For this review, take the finished solid that the model builds, in its own axes (mm). Give positions to 0.01 mm unless a question says otherwise; leave off trailing zeros. Write each loop counter-clockwise with the first axis right and the second up, starting at its lowest first coordinate (ties: lowest second). Pieces come first, ordered by that corner, then holes.
Q1. Insertion check: P1, Ø5, axis at x = 108, z = -27, coming from the -Y side; P2, Ø1.9, axis at x = -215, z = -181.4, coming from the +Y side. Each pin has a flat end and moves straight along its axis. Give the tip position at first contact, or say it passes through.
Q2. We need section A-A (x = -107.5). Write out the cut boundary in (y, z), then the cut area to 3 significant figures.
Q3. For line 1 (Z direction, x = -215, y = 0.6); line 2 (X direction, y = 0.6, z = -1.4); line 3 (X direction, y = 0.65, z = 188.6), list the stretches that pass through material, from the lowest coordinate up.
```python
from build123d import *

# Parameters (mm, degrees)
CROQUIS1_W              = 455
CROQUIS1_H              = 409
SALIENTE_EXTRUIR1_DEPTH = 1
CORTAR_EXTRUIR1_REACH   = 307.904
CROQUIS2_R              = 1.6
CORTAR_EXTRUIR2_REACH   = 307.904
CROQUIS3_R              = 5
CORTAR_EXTRUIR3_REACH   = 307.904
CROQUIS4_R              = 1.6
MOVER_CARA1_BY          = 5
CORTAR_EXTRUIR4_DEPTH   = 10


with BuildPart() as part:
    # Croquis1 → Saliente-Extruir1 (new body)
    with BuildSketch(Plane(origin=(0, 0, 0), x_dir=(1, 0, 0), z_dir=(0, 1, 0))):
        Rectangle(CROQUIS1_W, CROQUIS1_H)
    extrude(amount=SALIENTE_EXTRUIR1_DEPTH)

    # Croquis2 → Cortar-Extruir1 (cut, up to next)
    with BuildSketch(Plane.XZ, mode=Mode.PRIVATE) as cortar_extruir1_sk1:
        with Locations(Location((-215, 178.6, 0), (0, 0, 270))):
            Circle(CROQUIS2_R)
    cortar_extruir1_tool1 = extrude(cortar_extruir1_sk1.sketch, amount=-CORTAR_EXTRUIR1_REACH, mode=Mode.PRIVATE) & part.part
    # Croquis2 → Cortar-Extruir1 (cut, up to next)
    with BuildSketch(Plane.XZ, mode=Mode.PRIVATE) as cortar_extruir1_sk2:
        with Locations(Location((-215, -181.4, 0), (0, 0, 270))):
            Circle(CROQUIS2_R)
    cortar_extruir1_tool2 = extrude(cortar_extruir1_sk2.sketch, amount=-CORTAR_EXTRUIR1_REACH, mode=Mode.PRIVATE) & part.part
    # Croquis2 → Cortar-Extruir1 (cut, up to next)
    with BuildSketch(Plane.XZ, mode=Mode.PRIVATE) as cortar_extruir1_sk3:
        with Locations(Location((215, -181.4, 0), (0, 0, 270))):
            Circle(CROQUIS2_R)
    cortar_extruir1_tool3 = extrude(cortar_extruir1_sk3.sketch, amount=-CORTAR_EXTRUIR1_REACH, mode=Mode.PRIVATE) & part.part
    # Croquis2 → Cortar-Extruir1 (cut, up to next)
    with BuildSketch(Plane.XZ, mode=Mode.PRIVATE) as cortar_extruir1_sk4:
        with Locations(Location((215, 178.6, 0), (0, 0, 270))):
            Circle(CROQUIS2_R)
    cortar_extruir1_tool4 = extrude(cortar_extruir1_sk4.sketch, amount=-CORTAR_EXTRUIR1_REACH, mode=Mode.PRIVATE) & part.part
    # Croquis2 → Cortar-Extruir1 (cut, up to next)
    with BuildSketch(Plane.XZ, mode=Mode.PRIVATE) as cortar_extruir1_sk5:
        with Locations(Location((0, 31.25, 0), (0, 0, 270))):
            Circle(CROQUIS2_R)
    cortar_extruir1_tool5 = extrude(cortar_extruir1_sk5.sketch, amount=-CORTAR_EXTRUIR1_REACH, mode=Mode.PRIVATE) & part.part
    add(cortar_extruir1_tool1.solids().sort_by_distance((-215, 0, 178.6))[0], mode=Mode.SUBTRACT)
    add(cortar_extruir1_tool2.solids().sort_by_distance((-215, 0, -181.4))[0], mode=Mode.SUBTRACT)
    add(cortar_extruir1_tool3.solids().sort_by_distance((215, 0, -181.4))[0], mode=Mode.SUBTRACT)
    add(cortar_extruir1_tool4.solids().sort_by_distance((215, 0, 178.6))[0], mode=Mode.SUBTRACT)
    add(cortar_extruir1_tool5.solids().sort_by_distance((0, 0, 31.25))[0], mode=Mode.SUBTRACT)

    # Croquis3 → Cortar-Extruir2 (cut, up to next)
    with BuildSketch(Plane.XZ, mode=Mode.PRIVATE) as cortar_extruir2_sk1:
        with Locations(Location((-157.5, 38.6, 0), (0, 0, 270))):
            Circle(CROQUIS3_R)
    cortar_extruir2_tool1 = extrude(cortar_extruir2_sk1.sketch, amount=-CORTAR_EXTRUIR2_REACH, mode=Mode.PRIVATE) & part.part
    # Croquis3 → Cortar-Extruir2 (cut, up to next)
    with BuildSketch(Plane.XZ, mode=Mode.PRIVATE) as cortar_extruir2_sk2:
        with Locations(Location((-107.5, 38.6, 0), (0, 0, 270))):
            Circle(CROQUIS3_R)
    cortar_extruir2_tool2 = extrude(cortar_extruir2_sk2.sketch, amount=-CORTAR_EXTRUIR2_REACH, mode=Mode.PRIVATE) & part.part
    # Croquis3 → Cortar-Extruir2 (cut, up to next)
    with BuildSketch(Plane.XZ, mode=Mode.PRIVATE) as cortar_extruir2_sk3:
        with Locations(Location((-107.5, 188.6, 0), (0, 0, 270))):
            Circle(CROQUIS3_R)
    cortar_extruir2_tool3 = extrude(cortar_extruir2_sk3.sketch, amount=-CORTAR_EXTRUIR2_REACH, mode=Mode.PRIVATE) & part.part
    # Croquis3 → Cortar-Extruir2 (cut, up to next)
    with BuildSketch(Plane.XZ, mode=Mode.PRIVATE) as cortar_extruir2_sk4:
        with Locations(Location((-157.5, 188.6, 0), (0, 0, 270))):
            Circle(CROQUIS3_R)
    cortar_extruir2_tool4 = extrude(cortar_extruir2_sk4.sketch, amount=-CORTAR_EXTRUIR2_REACH, mode=Mode.PRIVATE) & part.part
    add(cortar_extruir2_tool1.solids().sort_by_distance((-157.5, 0, 38.6))[0], mode=Mode.SUBTRACT)
    add(cortar_extruir2_tool2.solids().sort_by_distance((-107.5, 0, 38.6))[0], mode=Mode.SUBTRACT)
    add(cortar_extruir2_tool3.solids().sort_by_distance((-107.5, 0, 188.6))[0], mode=Mode.SUBTRACT)
    add(cortar_extruir2_tool4.solids().sort_by_distance((-157.5, 0, 188.6))[0], mode=Mode.SUBTRACT)

    # Croquis4 → Cortar-Extruir3 (cut, up to next)
    with BuildSketch(Plane.XZ, mode=Mode.PRIVATE) as cortar_extruir3_sk1:
        with Locations(Location((-215, -1.4, 0), (0, 0, 270))):
            Circle(CROQUIS4_R)
    cortar_extruir3_tool1 = extrude(cortar_extruir3_sk1.sketch, amount=-CORTAR_EXTRUIR3_REACH, mode=Mode.PRIVATE) & part.part
    # Croquis4 → Cortar-Extruir3 (cut, up to next)
    with BuildSketch(Plane.XZ, mode=Mode.PRIVATE) as cortar_extruir3_sk2:
        with Locations(Location((215, -1.4, 0), (0, 0, 270))):
            Circle(CROQUIS4_R)
    cortar_extruir3_tool2 = extrude(cortar_extruir3_sk2.sketch, amount=-CORTAR_EXTRUIR3_REACH, mode=Mode.PRIVATE) & part.part
    # Croquis4 → Cortar-Extruir3 (cut, up to next)
    with BuildSketch(Plane.XZ, mode=Mode.PRIVATE) as cortar_extruir3_sk3:
        with Locations(Location((0, 188.6, 0), (0, 0, 270))):
            Circle(CROQUIS4_R)
    cortar_extruir3_tool3 = extrude(cortar_extruir3_sk3.sketch, amount=-CORTAR_EXTRUIR3_REACH, mode=Mode.PRIVATE) & part.part
    # Croquis4 → Cortar-Extruir3 (cut, up to next)
    with BuildSketch(Plane.XZ, mode=Mode.PRIVATE) as cortar_extruir3_sk4:
        with Locations(Location((30, -181.4, 0), (0, 0, 270))):
            Circle(CROQUIS4_R)
    cortar_extruir3_tool4 = extrude(cortar_extruir3_sk4.sketch, amount=-CORTAR_EXTRUIR3_REACH, mode=Mode.PRIVATE) & part.part
    add(cortar_extruir3_tool1.solids().sort_by_distance((-215, 0, -1.4))[0], mode=Mode.SUBTRACT)
    add(cortar_extruir3_tool2.solids().sort_by_distance((215, 0, -1.4))[0], mode=Mode.SUBTRACT)
    add(cortar_extruir3_tool3.solids().sort_by_distance((0, 0, 188.6))[0], mode=Mode.SUBTRACT)
    add(cortar_extruir3_tool4.solids().sort_by_distance((30, 0, -181.4))[0], mode=Mode.SUBTRACT)

    # Mover cara1: a face moved inward by 5.0
    extrude(part.faces().sort_by_distance((0, 0.5, -204.5))[0], amount=MOVER_CARA1_BY, dir=(0, 0, 1), mode=Mode.SUBTRACT)

    # Croquis5 → Cortar-Extruir4 (cut)
    with BuildSketch(Plane.XZ):
        with BuildLine():
            Line((-162.5, 173.6), (-162.5, 188.6))
            ThreePointArc((-162.5, 188.6), (-157.5, 193.6), (-152.5, 188.6))
            Line((-152.5, 188.6), (-152.5, 173.6))
            ThreePointArc((-152.5, 173.6), (-157.5, 168.6), (-162.5, 173.6))
        make_face()
        with BuildLine():
            Line((-112.5, 173.6), (-112.5, 188.6))
            ThreePointArc((-112.5, 188.6), (-107.5, 193.6), (-102.5, 188.6))
            Line((-102.5, 188.6), (-102.5, 173.6))
            ThreePointArc((-102.5, 173.6), (-107.5, 168.6), (-112.5, 173.6))
        make_face()
        with BuildLine():
            Line((-162.5, 23.6), (-162.5, 38.6))
            ThreePointArc((-162.5, 38.6), (-157.5, 43.6), (-152.5, 38.6))
            Line((-152.5, 38.6), (-152.5, 23.6))
            ThreePointArc((-152.5, 23.6), (-157.5, 18.6), (-162.5, 23.6))
        make_face()
        with BuildLine():
            Line((-112.5, 23.6), (-112.5, 38.6))
            ThreePointArc((-112.5, 38.6), (-107.5, 43.6), (-102.5, 38.6))
            Line((-102.5, 38.6), (-102.5, 23.6))
            ThreePointArc((-102.5, 23.6), (-107.5, 18.6), (-112.5, 23.6))
        make_face()
    extrude(amount=-CORTAR_EXTRUIR4_DEPTH, mode=Mode.SUBTRACT)


solid = part.part
```
Computed:
1. P1: stops at y = 0
1. P2: passes through
2. outline: (0, -199.5) - (1, -199.5) - (1, 18.6) - (0, 18.6) - close; (0, 43.6) - (1, 43.6) - (1, 168.6) - (0, 168.6) - close; (0, 193.6) - (1, 193.6) - (1, 204.5) - (0, 204.5) - close
2. area: 354 mm2
3. line 1: z = -199.5 to -183, -179.8 to -3, 0.2 to 177, 180.2 to 204.5
3. line 2: x = -227.5 to -216.6, -213.4 to 213.4, 216.6 to 227.5
3. line 3: x = -227.5 to -162.5, -152.5 to -112.5, -102.5 to -1.6, 1.6 to 227.5
